Answer from the drawing. Dimensions are ordinates in mm from the lowest x, y and z of the part. Round coordinates to 2 decimals unless told otherwise and drop trailing zeros. Order: outer loops, then holes, each group sorted by start corner. A loop starts at its lowest first (then second) coordinate and runs counter-clockwise, first axis right, second up.
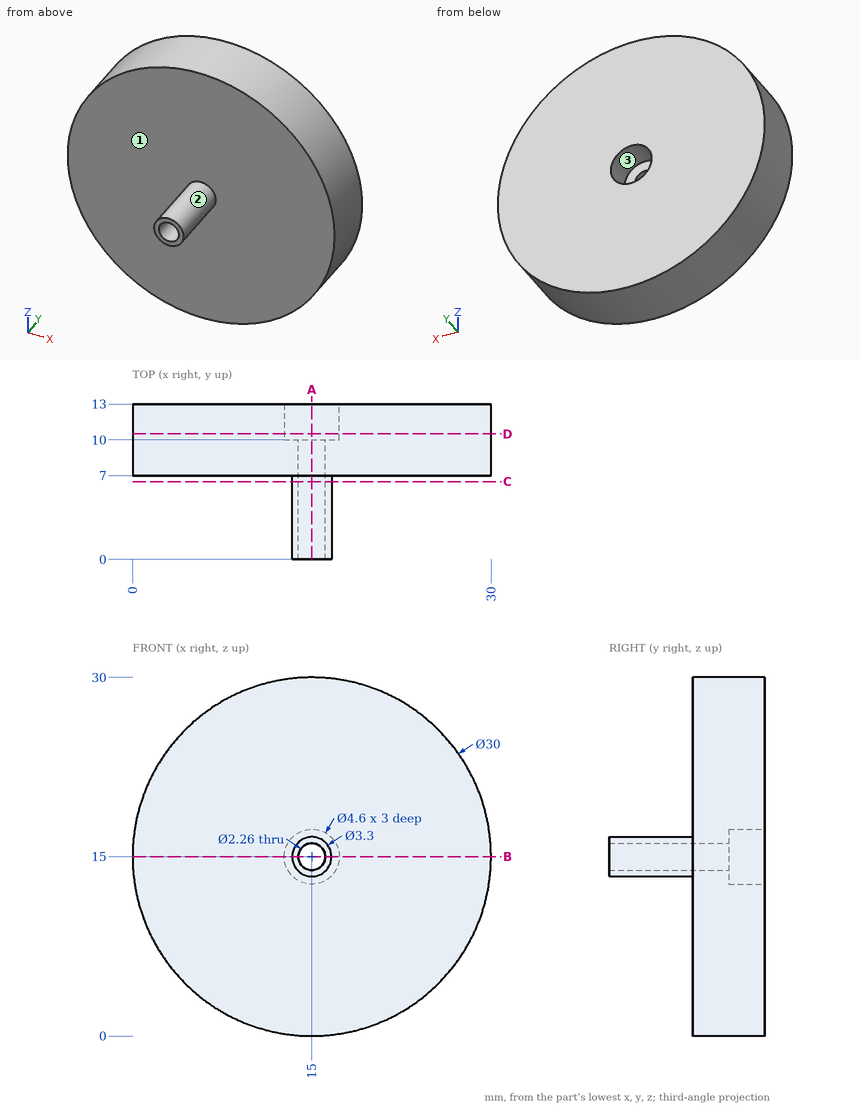
Q1. A cutting plane is placed at B-B, the plane z = 15. Give the vertices of the cut face in (x, y).
Outcome:
outline: (0, 7) - (13.35, 7) - (13.35, 0) - (13.87, 0) - (13.87, 10) - (12.7, 10) - (12.7, 13) - (0, 13) - close; (16.13, 0) - (16.65, 0) - (16.65, 7) - (30, 7) - (30, 13) - (17.3, 13) - (17.3, 10) - (16.13, 10) - close
Q2. A cutting plane is placed at D-D, the plane y = 10.5. Give the vertices of the cut face in (x, z), plus the area to 3 significant figures.
Outcome:
outline: circle Ø30 at (15, 15); hole circle Ø4.6 at (15, 15)
area: 690 mm2
Q3. For a pull along Z with two mould halves and no side action, classify the marked faces 1, 2 and 3 as released by +Z, released by -Z, zero draft, split by the parting line, or undercut.
Outcome:
face 1: zero draft
face 2: split by the parting line
face 3: undercut
Q4. Straight lines are drawn through the part: probe 1 along Z at (x, y) = (15, 6.75); probe 2 along Z at (x, y) = (15, 12.15); probe 3 along Y at (x, z) = (11, 20.5). For each, find the intervals that lie inside material, in ascending order.
Outcome:
probe 1: z = 13.35 to 13.87, 16.13 to 16.65
probe 2: z = 0 to 12.7, 17.3 to 30
probe 3: y = 7 to 13
Q5. Flat-ended cylindrical pins translate along their axes: pin 1 (1.5 mm diameter, centred on y = 8, z = 19.5, fed in from -X); pin 2 (6 mm diameter, centred on x = 25, y = 11, fed in from -Z); pin 3 (2 mm diameter, centred on x = 10, y = 6.5, fed in from -Z); pin 4 (3 mm diameter, centred on y = 3, z = 10.5, fed in from -X). Find the tip coordinate at first contact, or state that the pin passes through.
Outcome:
pin 1: stops at x = 0.48
pin 2: stops at z = 1.73
pin 3: stops at z = 0.58
pin 4: passes through
Q6. A cutting plane is placed at A-A, the plane x = 15. Give the vertices of the cut face in (y, z).
Outcome:
outline: (0, 13.35) - (7, 13.35) - (7, 0) - (13, 0) - (13, 12.7) - (10, 12.7) - (10, 13.87) - (0, 13.87) - close; (0, 16.13) - (10, 16.13) - (10, 17.3) - (13, 17.3) - (13, 30) - (7, 30) - (7, 16.65) - (0, 16.65) - close
Q7. A cutting plane is placed at C-C, the plane y = 6.5. Give the vertices of the cut face in (x, z).
Outcome:
outline: circle Ø3.3 at (15, 15); hole circle Ø2.26 at (15, 15)
